Could you check a few things on this model? Use its own coordinates, in mm. Coordinates: 2 decimals unless noted, no trailing zeros. Order: outer loops, then holes, each group sorted by start corner. A loop starts at its lowest first (then second) coordinate and runs counter-clockwise, first axis right, second up. Notation, with made-up numbers: (-22, -16) - (8, -16) arc R32 cw to (8, 21) - close; hole circle Ø10 at (68, -22.75). An arc over 180 degrees is marked (long way). Answer as a JSON object with one key per item and string values. Group by question number.
(1) Imagine slicing it at C-C, the plane x = -3. Write out the boundary of the cut face in (y, z).
(2) Imagine slicing it at A-A, the plane x = 89. Write out the boundary of the cut face in (y, z).
(3) Please list where these lines run through material, in increasing order: probe 1 along X at (y, z) = (31.5, 0.1); probe 2 along Y at (x, z) = (75.5, 0.4); probe 3 along X at (y, z) = (79, -0.6).
(4) Imagine slicing it at B-B, the plane y = 58. Write out the boundary of the cut face in (x, z), and give its area (3 significant figures).
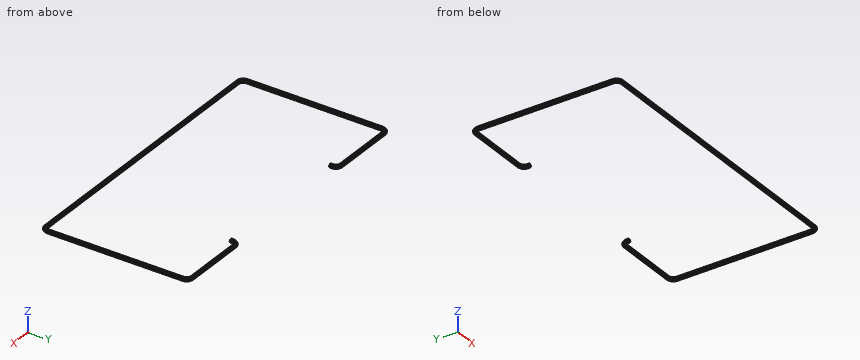
from build123d import *


with BuildPart() as f2:
    # F2: sweep along a path in F0
    with BuildLine(Plane.XY) as f2_path:
        Line((0, 0), (-97.79, 0))
        ThreePointArc((-97.79, 0), (-100.4840768363, 1.1159231637), (-101.6, 3.81))
        Line((-101.6, 3.81), (-101.6, 97.79))
        ThreePointArc((-101.6, 97.79), (-100.4840768363, 100.4840768363), (-97.79, 101.6))
        Line((-97.79, 101.6), (-54.61, 101.6))
        ThreePointArc((-54.61, 101.6), (-51.9159231637, 100.4840768363), (-50.8, 97.79))
        Line((-50.8, 97.79), (-50.8, 96.52))
    # F1 (on Right) → F2 (sweep)
    with BuildSketch(Plane.YZ):
        Polygon((0.7180774052, -1.0475041003), (1.145625325, -0.5481264588), (1.266203864, 0.0981212247), (1.0475041003, 0.7180774052), (0.5481264588, 1.145625325), (-0.0981212247, 1.266203864), (-0.7180774052, 1.0475041003), (-1.145625325, 0.5481264588), (-1.266203864, -0.0981212247), (-1.0475041003, -0.7180774052), (-0.5481264588, -1.145625325), (0.0981212247, -1.266203864), align=None)
    sweep(path=f2_path.line)

    # F3: F2 across plane


with BuildPart() as f2_1:
    add(f2.part)
    add(f2.part.mirror(Plane.YZ))


solid = f2_1.part
Result set:
{
 "1": {"outline": "(-1.27, -0.1) - (-1.05, -0.72) - (-0.55, -1.15) - (0.1, -1.27) - (0.72, -1.05) - (1.15, -0.55) - (1.27, 0.1) - (1.05, 0.72) - (0.55, 1.15) - (-0.1, 1.27) - (-0.72, 1.05) - (-1.15, 0.55) - close"},
 "2": {"outline": "(-1.27, -0.1) - (-1.05, -0.72) - (-0.55, -1.15) - (0.1, -1.27) - (0.72, -1.05) - (1.15, -0.55) - (1.27, 0.1) - (1.05, 0.72) - (0.55, 1.15) - (-0.1, 1.27) - (-0.72, 1.05) - (-1.15, 0.55) - close; (100.33, 0.1) - (100.45, -0.55) - (100.88, -1.05) - (101.5, -1.27) - (102.15, -1.15) - (102.65, -0.72) - (102.87, -0.1) - (102.75, 0.55) - (102.32, 1.05) - (101.7, 1.27) - (101.05, 1.15) - (100.55, 0.72) - close"},
 "3": {"probe 1": "x = -102.83 to -100.33, 100.33 to 102.83", "probe 2": "y = -1.17 to 1.16, 100.44 to 102.77", "probe 3": "x = -102.69 to -100.5, 100.5 to 102.69"},
 "4": {"outline": "(-102.87, -0.1) - (-102.65, -0.72) - (-102.15, -1.15) - (-101.5, -1.27) - (-100.88, -1.05) - (-100.45, -0.55) - (-100.33, 0.1) - (-100.55, 0.72) - (-101.05, 1.15) - (-101.7, 1.27) - (-102.32, 1.05) - (-102.75, 0.55) - close; (100.33, 0.1) - (100.45, -0.55) - (100.88, -1.05) - (101.5, -1.27) - (102.15, -1.15) - (102.65, -0.72) - (102.87, -0.1) - (102.75, 0.55) - (102.32, 1.05) - (101.7, 1.27) - (101.05, 1.15) - (100.55, 0.72) - close", "area": "9.68 mm^2"}
}
